```python
from build123d import *

# Parameters (mm, degrees)
BOSS_EXTRUDE1_DEPTH                     = 25
BOSS_EXTRUDE2_DEPTH                     = 10
CBORE_FOR_M8_HEX_HEAD_BOLT1_D           = 15
CBORE_FOR_M8_HEX_HEAD_BOLT1_CBORE_D     = 30
CBORE_FOR_M8_HEX_HEAD_BOLT1_CBORE_DEPTH = 10
BOSS_EXTRUDE3_DEPTH                     = 70
CUT_EXTRUDE1_DEPTH                      = 20
SKETCH7_R                               = 35.5
BOSS_EXTRUDE4_DEPTH                     = 130
SKETCH8_R                               = 20.5
CUT_EXTRUDE2_DEPTH                      = 224
SKETCH9_R                               = 38.333333333
BOSS_EXTRUDE5_DEPTH                     = 130
SKETCH10_R                              = 20.5
CUT_EXTRUDE3_DEPTH                      = 211
CHAMFER1_SIZE                           = 2


with BuildPart() as part:
    # Sketch1 → Boss-Extrude1 (new body)
    with BuildSketch(Plane.XY):
        with BuildLine():
            Line((10, 0), (190, 0))
            ThreePointArc((190, 0), (197.071067812, 2.928932188), (200, 10))
            Line((200, 10), (200, 203))
            ThreePointArc((200, 203), (197.071067812, 210.071067812), (190, 213))
            Line((190, 213), (10, 213))
            ThreePointArc((10, 213), (2.928932188, 210.071067812), (0, 203))
            Line((0, 203), (0, 10))
            ThreePointArc((0, 10), (2.928932188, 2.928932188), (10, 0))
        make_face()
    extrude(amount=BOSS_EXTRUDE1_DEPTH)

    # Sketch2 → Boss-Extrude2 (add)
    with BuildSketch(Plane.XY.offset(25)):
        with BuildLine():
            Line((200, 60), (200, 10))
            ThreePointArc((200, 10), (197.071067812, 2.928932188), (190, 0))
            Line((190, 0), (140, 0))
            Line((140, 0), (140, 45))
            ThreePointArc((140, 45), (144.393398282, 55.606601718), (155, 60))
            Line((155, 60), (200, 60))
        make_face()
    extrude(amount=BOSS_EXTRUDE2_DEPTH)

    # CBORE for M8 Hex Head Bolt1 (through all)
    with Locations(Plane.XY.offset(35)):
        with Locations((170, 30)):
            CounterBoreHole(CBORE_FOR_M8_HEX_HEAD_BOLT1_D / 2, CBORE_FOR_M8_HEX_HEAD_BOLT1_CBORE_D / 2, CBORE_FOR_M8_HEX_HEAD_BOLT1_CBORE_DEPTH)

    # Sketch5 → Boss-Extrude3 (add)
    with BuildSketch(Plane.XY.offset(25)):
        with BuildLine():
            Line((30, 0), (30, 80))
            ThreePointArc((30, 80), (93.639610307, 106.360389693), (120, 170))
            Line((120, 170), (200, 170))
            Line((200, 170), (200, 155))
            Line((200, 155), (133.923048454, 155))
            ThreePointArc((133.923048454, 155), (104.246212025, 95.753787975), (45, 66.076951546))
            Line((45, 66.076951546), (45, 0))
            Line((45, 0), (30, 0))
        make_face()
    extrude(amount=BOSS_EXTRUDE3_DEPTH)

    # Sketch6 → Cut-Extrude1 (cut)
    with BuildSketch(Plane.XY.offset(25)):
        with BuildLine():
            Line((54, 50.752358514), (54, 19))
            ThreePointArc((54, 19), (56.928932188, 11.928932188), (64, 9))
            Line((64, 9), (121, 9))
            ThreePointArc((121, 9), (128.071067812, 11.928932188), (131, 19))
            Line((131, 19), (131, 45))
            ThreePointArc((131, 45), (138.029437252, 61.970562748), (155, 69))
            Line((155, 69), (181, 69))
            ThreePointArc((181, 69), (188.071067812, 71.928932188), (191, 79))
            Line((191, 79), (191, 136))
            ThreePointArc((191, 136), (188.071067812, 143.071067812), (181, 146))
            Line((181, 146), (149.247641486, 146))
            ThreePointArc((149.247641486, 146), (143.223496519, 143.981834214), (139.630896205, 138.741935484))
            ThreePointArc((139.630896205, 138.741935484), (110.610173055, 89.389826945), (61.258064516, 60.369103795))
            ThreePointArc((61.258064516, 60.369103795), (56.018165786, 56.776503481), (54, 50.752358514))
        make_face()
    extrude(amount=-CUT_EXTRUDE1_DEPTH, mode=Mode.SUBTRACT)

    # Sketch7 → Boss-Extrude4 (add)
    with BuildSketch(Plane(origin=(0, -10, 0), x_dir=(-1, 0, 0), z_dir=(0, -1, 0))):
        with Locations((-37.5, -95)):
            Circle(SKETCH7_R)
    extrude(amount=-BOSS_EXTRUDE4_DEPTH)

    # Sketch8 → Cut-Extrude2 (cut, through all)
    with BuildSketch(Plane.XZ.offset(10)):
        with Locations((37.5, 95)):
            Circle(SKETCH8_R)
    extrude(amount=-CUT_EXTRUDE2_DEPTH, mode=Mode.SUBTRACT)

    # Sketch9 → Boss-Extrude5 (add)
    with BuildSketch(Plane(origin=(210, 0, 0), x_dir=(0, 0, -1), z_dir=(1, 0, 0))):
        with Locations((-95, 162.5)):
            Circle(SKETCH9_R)
    extrude(amount=-BOSS_EXTRUDE5_DEPTH)

    # Sketch10 → Cut-Extrude3 (cut, through all)
    with BuildSketch(Plane(origin=(210, 0, 0), x_dir=(0, 0, -1), z_dir=(1, 0, 0))):
        with Locations((-95, 162.5)):
            Circle(SKETCH10_R)
    extrude(amount=-CUT_EXTRUDE3_DEPTH, mode=Mode.SUBTRACT)

    # Chamfer1
    chamfer1_edges = [part.edges().sort_by_distance(p)[0] for p in [
        (17, 120, 95),
        (17, -10, 95),
        (80, 162.5, 115.5),
        (210, 162.5, 115.5),
    ]]
    chamfer(chamfer1_edges, length=CHAMFER1_SIZE)


solid = part.part
```
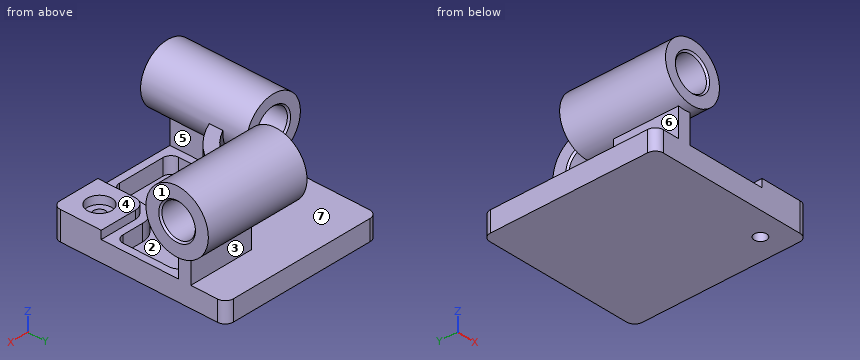
Read the model definition and answer for the solid it produces. Units are mm, in the model's axes. Face numbers are marked on the shaded views. A direction names the side the tool comes from. Round coordinates to 2 decimals unless told otherwise and drop trailing zeros. Write each loop counter-clockwise with the first axis right and the second up, starting at its lowest first coordinate (ties: lowest second). Pieces come first, ordered by that corner, then holes. Notation, with made-up numbers: (12.5, 59.5) -> (65.5, 59.5) arc R18 cw to (65.5, 93.5) -> close; hole circle Ø11 at (15.5, -12.75). An arc over 180 degrees is marked (long way). Answer in a Markdown table with one row per item. Add a question column.
1) Consider line 1 (Y direction, x = 170, z = 28); line 2 (Y direction, x = 170, z = 5.5); line 3 (X direction, y = 114.5, z = 89.5). Determine where each line is inside the solid, lowest interval first.
2) Find section A-A, the plane z = 29.5. Determine the outline of the cut face in (x, y), and give its area (3 significant figures).
3) Find section C-C, the plane y = 30. Determine the outline of the cut face in (x, z), and give its area (3 significant figures).
4) Determine the mould class of the marked faces 1, 2 and 3 for opening direction Y: pulls with the +Y half, pulls with the -Y half, needs draft (parallel to the pull), parting line crosses it, or undercut.
5) Find section D-D, the plane x = 37.5. Determine the outline of the cut face in (y, z), and give its area (3 significant figures).
6) Find section B-B, the plane x = 170. Determine the outline of the cut face in (y, z).
7) Which of the six approach directions +Z, -Z, +X, -X, +Y, -Y give full straight-line access (tool end or side, diameter ignored) to the marked faces 4, 5, 6 and 7?
8) Given P1, Ø4, axis at x = 115, y = 27, coming from the +Z side; P2, Ø10, axis at x = 141.5, z = 71.5, coming from the -Y side; P3, Ø6, axis at x = 44, y = 121.5, coming from the +Z side, each flat-ended and moving along its own axis, determine where each tip first touches the part or whether it passes through.
Findings below:
| question | item | result |
|---|---|---|
| 1 | line 1 | 0 to 15, 45 to 60, 155 to 170 |
| 1 | line 2 | 0 to 22.5, 37.5 to 69, 146 to 213 |
| 1 | line 3 | 2.43 to 17.75, 57.25 to 72.57, 100.85 to 119.13 |
| 2 | outline | (30, 0) -> (45, 0) -> (45, 66.08) arc R105 ccw to (133.92, 155) -> (200, 155) -> (200, 170) -> (120, 170) arc R90 cw to (30, 80) -> close; (140, 0) -> (190, 0) arc R10 ccw to (200, 10) -> (200, 60) -> (155, 60) arc R15 ccw to (140, 45) -> close; hole circle Ø30 at (170, 30) |
| 2 | area | 7,080 mm² |
| 3 | outline | (0, 0) -> (162.5, 0) -> (162.5, 25) -> (155, 25) -> (155, 35) -> (140, 35) -> (140, 25) -> (131, 25) -> (131, 5) -> (54, 5) -> (54, 25) -> (45, 25) -> (45, 60.3) arc R35.5 ccw (long way) to (30, 60.3) -> (30, 25) -> (0, 25) -> close; (177.5, 0) -> (200, 0) -> (200, 35) -> (185, 35) -> (185, 25) -> (177.5, 25) -> close; hole circle Ø41 at (37.5, 95) |
| 3 | area | 6,550 mm² |
| 4 | face 1 | needs draft |
| 4 | face 2 | undercut |
| 4 | face 3 | pulls with the +Y half |
| 5 | outline | (-10, 59.5) -> (0, 59.5) -> (0, 0) -> (213, 0) -> (213, 25) -> (80.31, 25) -> (80.31, 59.5) -> (120, 59.5) -> (120, 72.5) -> (118, 74.5) -> (-8, 74.5) -> (-10, 72.5) -> close; (-10, 117.5) -> (-8, 115.5) -> (118, 115.5) -> (120, 117.5) -> (120, 130.5) -> (-10, 130.5) -> close |
| 5 | area | 12,000 mm² |
| 6 | outline | (0, 0) -> (22.5, 0) -> (22.5, 25) -> (15, 25) -> (15, 35) -> (0, 35) -> close; (37.5, 0) -> (213, 0) -> (213, 25) -> (170, 25) -> (170, 57.41) arc R38.33 ccw (long way) to (155, 57.41) -> (155, 25) -> (146, 25) -> (146, 5) -> (69, 5) -> (69, 25) -> (60, 25) -> (60, 35) -> (45, 35) -> (45, 25) -> (37.5, 25) -> close; hole circle Ø41 at (162.5, 95) |
| 7 | face 4 | +Z, +X, -Y |
| 7 | face 5 | -Y |
| 7 | face 6 | -X, +Y, -Y |
| 7 | face 7 | -X, +Y |
| 8 | P1 | z = 5 |
| 8 | P2 | y = 128.93 |
| 8 | P3 | z = 130.28 |
